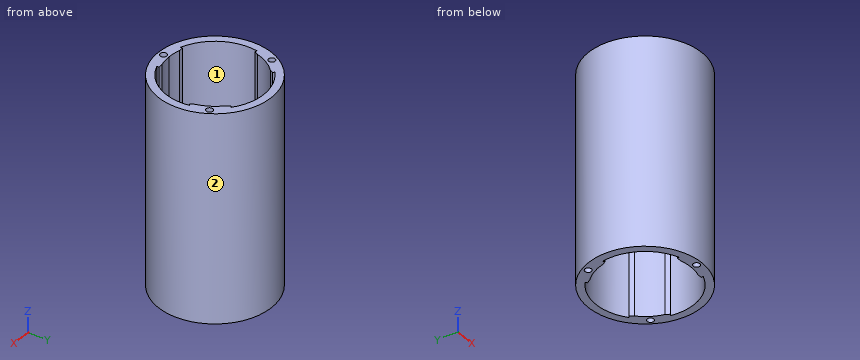
from build123d import *

# Parameters (mm, degrees)
F0_R     = 26
F0_R_2   = 1.5
F1_DEPTH = 95


with BuildPart() as f1:
    # F0 (on Top) → F1 (new body)
    with BuildSketch(Plane.XY):
        Circle(F0_R)
        with Locations((0, -23.5)):
            Circle(F0_R_2, mode=Mode.SUBTRACT)
        with Locations((-20.3515969889, 11.75)):
            Circle(F0_R_2, mode=Mode.SUBTRACT)
        with BuildLine():
            ThreePointArc((22.1726827981, 3.8238903663), (19.4855715851, -11.25), (7.7747552005, -21.1140517564))
            Line((7.7747552005, -21.1140517564), (7.7747552005, -20.1896557547))
            Line((7.7747552005, -20.1896557547), (5.7773523787, -20.1896557547))
            ThreePointArc((5.7773523787, -20.1896557547), (2.9169529609, -20.7964272274), (0, -21))
            ThreePointArc((0, -21), (-2.9169529609, -20.7964272274), (-5.7773523787, -20.1896557547))
            Line((-5.7773523787, -20.1896557547), (-7.7747552005, -20.1896557547))
            Line((-7.7747552005, -20.1896557547), (-7.7747552005, -21.1140517564))
            ThreePointArc((-7.7747552005, -21.1140517564), (-19.4855715851, -11.25), (-22.1726827981, 3.8238903663))
            Line((-22.1726827981, 3.8238903663), (-21.3721323775, 3.3616923655))
            Line((-21.3721323775, 3.3616923655), (-20.3734309666, 5.0914939507))
            ThreePointArc((-20.3734309666, 5.0914939507), (-18.1896766972, 10.5018147376), (-14.5960785878, 15.0981618039))
            Line((-14.5960785878, 15.0981618039), (-13.5973771769, 16.8279633892))
            Line((-13.5973771769, 16.8279633892), (-14.3979275976, 17.2901613901))
            ThreePointArc((-14.3979275976, 17.2901613901), (0, 22.5), (14.3979275976, 17.2901613901))
            Line((14.3979275976, 17.2901613901), (13.5973771769, 16.8279633892))
            Line((13.5973771769, 16.8279633892), (14.5960785878, 15.0981618039))
            ThreePointArc((14.5960785878, 15.0981618039), (18.2034997005, 10.5097954523), (20.3734309666, 5.0914939507))
            Line((20.3734309666, 5.0914939507), (21.3721323775, 3.3616923655))
            Line((21.3721323775, 3.3616923655), (22.1726827981, 3.8238903663))
        make_face(mode=Mode.SUBTRACT)
        with Locations((20.3515969889, 11.75)):
            Circle(F0_R_2, mode=Mode.SUBTRACT)
    extrude(amount=F1_DEPTH)


solid = f1.part
Check sheet for the modelled part. Datum: model origin and axes. Units: mm. Face numbers are marked on the shaded views. Round coordinates to 2 decimals unless told otherwise and drop trailing zeros. Order: outer loops, then holes, each group sorted by start corner. A loop starts at its lowest first (then second) coordinate and runs counter-clockwise, first axis right, second up. Notation, with made-up numbers: M -37.75,-9 L 2.25,-9 A26 cw 2.25,27 Z; hole C -29,-31.75 d6. An arc over 180 degrees is marked long. One line per item, written item: value. Start each with the question number.
1. Section check B-B on x = 12.5. Enter the section's corners in (y, z), and give its area (3 significant figures).
2. Scan lines: line 1 along X through (y, z) = (13, 30); line 2 along Y through (x, z) = (-19, 25.5); line 3 along X through (y, z) = (11, 42). Record each from-to range of solid material in increasing order.
3. Section check A-A on y = 1. Enter the section's corners in (x, z), and give its area (3 significant figures).
4. Section check D-D on y = 11.75. Enter the section's corners in (x, z), and give its area (3 significant figures).
5. Release check for a two-part mould opening along X. For the marked faces 1 and 2 record: released by +X, released by -X, zero draft, split by the parting line, or undercut.
6. Gauge pin test, flat ends, axial feed: P1, Ø10, axis at y = -17, z = 61.5, coming from the -X side; P2, Ø2, axis at x = 7, z = 28.5, coming from the +Y side; P3, Ø1, axis at y = -17, z = 26.5, coming from the -X side; P4, Ø2, axis at x = 19.5, y = 2, coming from the +Z side. Record the tip position at first contact, or that the pin passes through.
7. Section check C-C on z = 34. Enter the section's corners in (x, y), and give its area (3 significant figures).
Results found:
1. outline: M -22.8,0 L -18.71,0 L -18.71,95 L -22.8,95 Z; M 18.71,0 L 22.8,0 L 22.8,95 L 18.71,95 Z
1. area: 777 mm^2
2. line 1: -22.52 to -21.18, -19.52 to -16.5, 16.51 to 19.52, 21.18 to 22.52
2. line 2: -17.75 to -12.05, 8.95 to 11.1, 12.4 to 17.75
2. line 3: -23.56 to -21.65, -19.05 to -17.89, 17.91 to 19.05, 21.65 to 23.56
3. outline: M -25.98,0 L -22.48,0 L -22.48,95 L -25.98,95 Z; M 22.48,0 L 25.98,0 L 25.98,95 L 22.48,95 Z
3. area: 666 mm^2
4. outline: M -23.19,0 L -21.85,0 L -21.85,95 L -23.19,95 Z; M -18.85,0 L -17.41,0 L -17.41,95 L -18.85,95 Z; M 17.43,0 L 18.85,0 L 18.85,95 L 17.43,95 Z; M 21.85,0 L 23.19,0 L 23.19,95 L 21.85,95 Z
4. area: 527 mm^2
5. face 1: undercut
5. face 2: split by the parting line
6. P1: x = -23.07
6. P2: y = 25.3
6. P3: x = -20.09
6. P4: through
7. outline: C 0,0 d52; hole M -22.17,3.82 A22.5 ccw -7.77,-21.11 L -7.77,-20.19 L -5.78,-20.19 A21 ccw 5.78,-20.19 L 7.77,-20.19 L 7.77,-21.11 A22.5 ccw 22.17,3.82 L 21.37,3.36 L 20.37,5.09 A20.52 ccw 14.6,15.1 L 13.6,16.83 L 14.4,17.29 A22.5 ccw -14.4,17.29 L -13.6,16.83 L -14.6,15.1 A20.91 ccw -20.37,5.09 L -21.37,3.36 Z; hole C -20.35,11.75 d3; hole C 0,-23.5 d3; hole C 20.35,11.75 d3
7. area: 580 mm^2
